Geometry: final body of the model. Coordinates: model frame, mm. Face numbers are marked on the shaded views. A direction names the side the tool comes from. Give positions to 0.01 mm unless a question says otherwise; leave off trailing zeros. Write each loop counter-clockwise with the first axis right and the second up, starting at its lowest first coordinate (ties: lowest second). Pieces come first, ordered by that corner, then holes. Notation, with made-up numbers: (41, 86.25) -> (92, 86.25) arc R23 ccw to (92, 116.25) -> close; hole circle Ø4 at (-25.5, -5). An arc over 180 degrees is marked (long way). Answer as a JSON object with one key per item and string values.
from build123d import *

# Parameters (mm, degrees)
SKETCH1_W                      = 30
SKETCH1_H                      = 10
BOSS_EXTRUDE1_DEPTH            = 200
SKETCH2_W                      = 30
SKETCH2_H                      = 25
BOSS_EXTRUDE2_DEPTH            = 30
SKETCH3_R                      = 14
CUT_EXTRUDE1_DEPTH             = 23
FILLET1_R                      = 10
FILLET2_R                      = 10
SKETCH5_W                      = 30
SKETCH5_H                      = 25
BOSS_EXTRUDE3_DEPTH            = 30
SKETCH6_R                      = 14
CUT_EXTRUDE2_DEPTH             = 30
FILLET3_R                      = 10
FILLET4_R                      = 10
CBORE_FOR_M3_SHCS1_D           = 3.4
CBORE_FOR_M3_SHCS1_CBORE_D     = 5.4
CBORE_FOR_M3_SHCS1_CBORE_DEPTH = 3
SKETCH11_R                     = 10
CUT_EXTRUDE3_DEPTH             = 10


with BuildPart() as part:
    # Sketch1 → Boss-Extrude1 (new body)
    with BuildSketch(Plane(origin=(0, 0, 0), x_dir=(1, 0, 0), z_dir=(0, 1, 0))):
        Rectangle(SKETCH1_W, SKETCH1_H)
    extrude(amount=BOSS_EXTRUDE1_DEPTH)

    # Sketch2 → Boss-Extrude2 (add)
    with BuildSketch(Plane.XY.offset(5)):
        with Locations((0, 12.5)):
            Rectangle(SKETCH2_W, SKETCH2_H)
    extrude(amount=BOSS_EXTRUDE2_DEPTH)

    # Sketch3 → Cut-Extrude1 (cut)
    with BuildSketch(Plane(origin=(0, 25, 0), x_dir=(1, 0, 0), z_dir=(0, 1, 0))):
        with Locations(Location((0, -20, 0), (0, 0, 270))):
            Circle(SKETCH3_R)
    extrude(amount=-CUT_EXTRUDE1_DEPTH, mode=Mode.SUBTRACT)

    # Fillet1
    fillet1_edges = [part.edges().sort_by_distance(p)[0] for p in [
        (15, 12.5, 35),
    ]]
    fillet(fillet1_edges, radius=FILLET1_R)

    # Fillet2
    fillet2_edges = [part.edges().sort_by_distance(p)[0] for p in [
        (-15, 12.5, 35),
    ]]
    fillet(fillet2_edges, radius=FILLET2_R)

    # Sketch5 → Boss-Extrude3 (add)
    with BuildSketch(Plane.XY.offset(5)):
        with Locations((0, 159.428426998)):
            Rectangle(SKETCH5_W, SKETCH5_H)
    extrude(amount=BOSS_EXTRUDE3_DEPTH)

    # Sketch6 → Cut-Extrude2 (cut)
    with BuildSketch(Plane(origin=(0, 171.928426998, 0), x_dir=(1, 0, 0), z_dir=(0, 1, 0))):
        with Locations(Location((0, -20, 0), (0, 0, 270))):
            Circle(SKETCH6_R)
    extrude(amount=-CUT_EXTRUDE2_DEPTH, mode=Mode.SUBTRACT)

    # Fillet3
    fillet3_edges = [part.edges().sort_by_distance(p)[0] for p in [
        (-15, 159.428426998, 35),
    ]]
    fillet(fillet3_edges, radius=FILLET3_R)

    # Fillet4
    fillet4_edges = [part.edges().sort_by_distance(p)[0] for p in [
        (15, 159.428426998, 35),
    ]]
    fillet(fillet4_edges, radius=FILLET4_R)

    # CBORE for M3 SHCS1 (through all)
    with Locations(Plane.XY.offset(5)):
        with Locations((-7.5, 192.982106749)):
            cbore_for_m3_shcs1 = CounterBoreHole(CBORE_FOR_M3_SHCS1_D / 2, CBORE_FOR_M3_SHCS1_CBORE_D / 2, CBORE_FOR_M3_SHCS1_CBORE_DEPTH)

    # Mirror1: CBORE for M3 SHCS1 across plane
    add(cbore_for_m3_shcs1.mirror(Plane(origin=(0, 0, 0), x_dir=(0, 0, 1), z_dir=(1, 0, 0))), mode=Mode.SUBTRACT)

    # Sketch11 → Cut-Extrude3 (cut)
    with BuildSketch(Plane(origin=(0, 2, 0), x_dir=(1, 0, 0), z_dir=(0, 1, 0))):
        with Locations(Location((0, -20, 0), (0, 0, 270))):
            Circle(SKETCH11_R)
    extrude(amount=-CUT_EXTRUDE3_DEPTH, mode=Mode.SUBTRACT)


solid = part.part
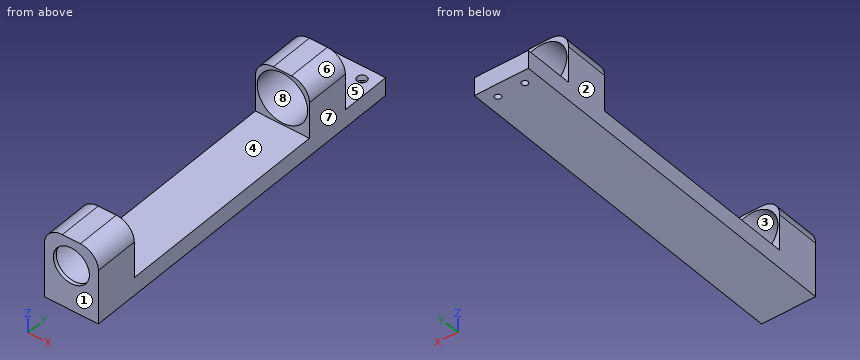
Q1. Cut plane C-C (x = 7.5). State how many separate pieces and enclosed holes the cut face has, and give its area (3 significant figures).
Values:
{"separate pieces": "4", "enclosed holes": "0", "area": "2,280 mm²"}
Q2. Cut plane A-A (x = 0). Return the cut outline in (y, z).
Values:
{"outline": "(0, -5) -> (200, -5) -> (200, 5) -> (171.93, 5) -> (171.93, 6) -> (146.93, 6) -> (146.93, 5) -> (25, 5) -> (25, 6) -> (2, 6) -> (2, 10) -> (0, 10) -> close; (0, 30) -> (2, 30) -> (2, 34) -> (25, 34) -> (25, 35) -> (0, 35) -> close; (146.93, 34) -> (171.93, 34) -> (171.93, 35) -> (146.93, 35) -> close"}
Q3. Mould query, pull axis Z, two halves, no side actions, for the marked faces 6, 7 and 8. Classes: pulls with the +Z half, pulls with the -Z half, needs draft (parallel to the pull), parting line crosses it, or undercut.
Values:
{"face 6": "pulls with the +Z half", "face 7": "needs draft", "face 8": "undercut"}
Q4. Set-up query: the marked faces 1, 2, 3, 4 and 5. Return all of +Z, -Z, +X, -X, +Y, -Y with unobstructed straight access to the full face (end or side cutting, diameter ignored); none if empty.
Values:
{"face 1": "+Z, -Z, +X, -X, -Y", "face 2": "+Z, -Z, -X, +Y, -Y", "face 3": "+Y", "face 4": "+Z, +X, -X", "face 5": "+Z, +X, -X, +Y"}
Q5. Cut plane B-B (z = 20). Return the cut outline in (x, y), and give its area (3 significant figures).
Values:
{"outline": "(-15, 0) -> (-10, 0) -> (-10, 2) -> (-14, 2) -> (-14, 25) -> (-15, 25) -> close; (-15, 146.93) -> (-14, 146.93) -> (-14, 171.93) -> (-15, 171.93) -> close; (10, 0) -> (15, 0) -> (15, 25) -> (14, 25) -> (14, 2) -> (10, 2) -> close; (14, 146.93) -> (15, 146.93) -> (15, 171.93) -> (14, 171.93) -> close", "area": "116 mm²"}
Q6. First-contact query: P1, Ø6, axis at x = 9.5, z = 18.5, coming from the +Y side; P2, Ø9, axis at x = -0.5, y = 105, coming from the +Z side; P3, Ø12, axis at x = 8, z = 16.5, coming from the +Y side. Flat tips, straight axial feed; report the tip coordinate or a pass-through.
Values:
{"P1": "y = 2", "P2": "z = 5", "P3": "y = 171.93"}
Q7. Cut plane D-D (y = 112.5). Return the cut outline in (x, z).
Values:
{"outline": "(-15, -5) -> (15, -5) -> (15, 5) -> (-15, 5) -> close"}
Q8. Material intervals for L1, parallel to X at y = 153.75, z = 20; L2, parallel to Y at x = 7.5, z = 4.2; L3, parallel to Z at x = -12.5, y = 58.5, sorted ascending. Write a range as from..to.
Values:
{"L1": "-15..-14, 14..15", "L2": "0..190.28, 195.68..200", "L3": "-5..5"}
